Source: three-view drawing plus pictorial views. Frame: mm from the lowest corner of the part. A direction names the side the tool comes from. Coordinates: 2 decimals unless noted, no trailing zeros. Write each loop counter-clockwise with the first axis right and the second up, starting at its lowest first coordinate (ties: lowest second). Pieces come first, ordered by that corner, then holes. Notation, with made-up numbers: (17, 51) -> (50, 51) arc R14 cw to (50, 56) -> close; hole circle Ø5 at (32, -19.5). An arc over 180 degrees is marked (long way). One line per item, written item: value.
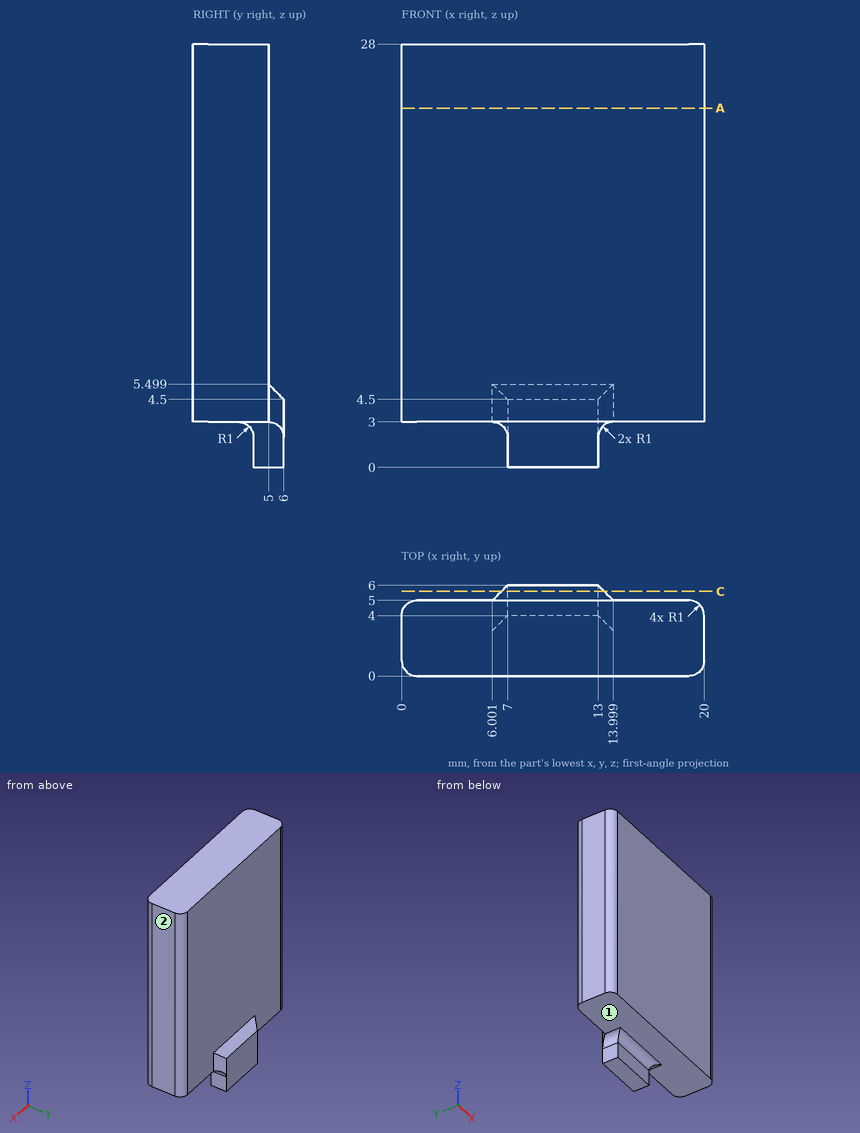
(1) Line query: line 1 (Y direction, x = 1.75, z = 16.75); line 2 (Z direction, x = 13, y = 0.9); line 3 (X direction, y = 4.3, z = 2.75) (1 decimal). Output: solid intervals per line, ascending. Write a range as [from, to].
Responses:
line 1: y = [0, 5]
line 2: z = [3, 28]
line 3: x = [6.7, 13.3]
(2) First-contact query: pin 1 (2 mm diameter, centred on x = 13.5, z = 23.5, fed in from +Y); pin 2 (2.5 mm diameter, centred on x = 14, y = 2, fed in from -Z); pin 3 (1 mm diameter, centred on y = 5.5, z = 2, fed in from +X) (1 decimal). Flat tips, straight axial feed; report the tip coordinate or a pass-through.
Responses:
pin 1: stops at y = 5
pin 2: stops at z = 2.97
pin 3: stops at x = 13.1
(3) Section C-C (y = 5.6). Return the cut outline in (x, z).
Responses:
outline: (6.6, 2.8) arc R1 cw to (7, 2) -> (7, 0) -> (13, 0) -> (13, 2) arc R1 cw to (13.4, 2.8) -> (13.4, 4.9) -> (6.6, 4.9) -> close
(4) Reachability of the marked faces 1 and 2 from +Z, -Z, +X, -X, +Y, -Y: full face, straight path, thin tool, end or side. Return the list, or none.
Responses:
face 1: -Z, -Y
face 2: +Z, -Z, +X, +Y, -Y
(5) Section A-A (z = 23.75). Return the cut outline in (x, y).
Responses:
outline: (0, 1) arc R1 ccw to (1, 0) -> (19, 0) arc R1 ccw to (20, 1) -> (20, 4) arc R1 ccw to (19, 5) -> (1, 5) arc R1 ccw to (0, 4) -> close
